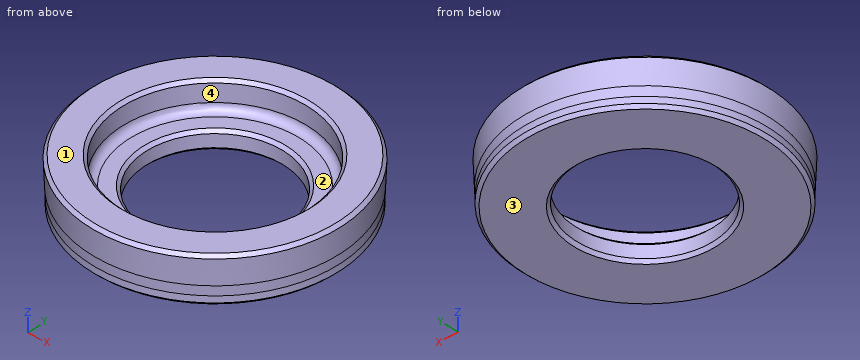
from build123d import *


# Not quite as in the source:
# - a fillet or chamfer that OpenCascade refuses, or shapes differently, is made with other operations: its cross-section is extruded or revolved along the edge and cut away or added


with BuildPart() as f1:
    # F0 (on Front) → F1 (revolve)
    with BuildSketch(Plane.XZ):
        with BuildLine():
            Line((-66.7483291848, 10), (-66.5397158787, 5))
            Line((-66.5397158787, 5), (-66.5397158787, 0))
            Line((-66.5397158787, 0), (-37, 0))
            Line((-37, 0), (-37, 10))
            Line((-37, 10), (-46, 10))
            ThreePointArc((-46, 10), (-48.8284271247, 11.1715728753), (-50, 14))
            Line((-50, 14), (-50, 25.0225278729))
            Line((-50, 25.0225278729), (-67.375109026, 25.0225278729))
            Line((-67.375109026, 25.0225278729), (-66.7483291848, 10))
        make_face()
    revolve(axis=Axis((0, 0, 30.7617206126), (0, 0, 1)))

    # F2: chamfer of 1.6 on 5 edges, made by hand

    # F2_s1 → F2_t2 (revolve, cut)
    with BuildSketch(Plane.XZ):
        Polygon((-38.6, 10), (-37, 8.4), (-37, 10), align=None)
    revolve(axis=Axis((0, 0, 10), (0, 0, 1)), mode=Mode.SUBTRACT)

    # F2_s3 → F2_t4 (revolve, cut)
    with BuildSketch(Plane.XZ):
        Polygon((-37, 1.6), (-38.6, 0), (-37, 0), align=None)
    revolve(axis=Axis((0, 0, 0), (0, 0, 1)), mode=Mode.SUBTRACT)

    # F2_s5 → F2_t6 (revolve, cut)
    with BuildSketch(Plane.XZ):
        Polygon((-64.9397158787, 0), (-66.5397158787, 1.6), (-66.5397158787, 0), align=None)
    revolve(axis=Axis((0, 0, 0), (0, 0, 1)), mode=Mode.SUBTRACT)

    # F2_s7 → F2_t8 (revolve, cut)
    with BuildSketch(Plane.XZ):
        Polygon((-51.6, 25.0225278729), (-50, 23.4225278729), (-50, 25.0225278729), align=None)
    revolve(axis=Axis((0, 0, 25.0225278729), (0, 0, 1)), mode=Mode.SUBTRACT)

    # F2_s9 → F2_t10 (revolve, cut)
    with BuildSketch(Plane.XZ):
        Polygon((-67.3055699404, 23.3558296431), (-65.7069607492, 25.0225278729), (-67.375109026, 25.0225278729), align=None)
    revolve(axis=Axis((0, 0, 25.0225278729), (0, 0, 1)), mode=Mode.SUBTRACT)


solid = f1.part
Work out the finished part from the listing and answer in its coordinate system (mm). Face numbers are marked on the shaded views. A direction names the side the tool comes from. Give positions to 0.01 mm unless a question says otherwise; leave off trailing zeros. Loops run counter-clockwise (first coordinate to the right, second up) from the corner with the lowest first, then second, coordinate; pieces in that order, holes last. Notation, with made-up numbers: (-29.75, 66.5) -> (27.25, 66.5) arc R17 ccw to (27.25, 96.5) -> close; hole circle Ø6 at (-8.75, 55). An arc over 180 degrees is marked (long way). Use a Markdown table: item, result. Add a question column.
1. Flat-ended cylindrical pins translate along their axes: pin 1 Ø1.5 at (x, y) = (-19, 31) entering from +Z; pin 2 Ø12 at (x, z) = (43.5, 4.5) entering from +Y; pin 3 Ø2 at (y, z) = (4, 11.5) entering from +X; pin 4 Ø12 at (x, y) = (-10.5, 43) entering from -Z. Find the tip coordinate at first contact, or state that the pin passes through.
2. Section B-B on z = 16.75 is taken. Determine the outline of the cut face in (x, y), and give its area (3 significant figures).
3. Section A-A on z = 6.75 is taken. Determine the outline of the cut face in (x, y), and give its area (3 significant figures).
4. For the marked faces 1 and 2, determine the directions among +Z, -Z, +X, -X, +Y, -Y from which every point of the face is accessible in a straight line to the end or side of a thin tool.
5. Determine the mould class of the marked faces 3 and 4 for opening direction X: released by +X, released by -X, zero draft, split by the parting line, or undercut.
6. Find the intervals of material crossed by probe 1 along Y at (x, z) = (0, 21.5); probe 2 along X at (y, z) = (0, 18); probe 3 along X at (y, z) = (11.5, 23.5), in increasing order.
Results below:
| question | item | result |
|---|---|---|
| 1 | pin 1 | stops at z = 8.51 |
| 1 | pin 2 | stops at y = 54.97 |
| 1 | pin 3 | stops at x = 66.76 |
| 1 | pin 4 | stops at z = 0 |
| 2 | outline | circle Ø134.06 at (0, 0); hole circle Ø100 at (0, 0) |
| 2 | area | 6,260 mm^2 |
| 3 | outline | circle Ø133.23 at (0, 0); hole circle Ø74 at (0, 0) |
| 3 | area | 9,640 mm^2 |
| 4 | face 1 | +Z, +X, -X, +Y, -Y |
| 4 | face 2 | +Z |
| 5 | face 3 | zero draft |
| 5 | face 4 | undercut |
| 6 | probe 1 | y = -67.23 to -50, 50 to 67.23 |
| 6 | probe 2 | x = -67.08 to -50, 50 to 67.08 |
| 6 | probe 3 | x = -66.18 to -48.74, 48.74 to 66.18 |
